Autodesk Inventor part; units mm, degrees
ref_plane "YZ Plane" through (0, 0, 0) normal (1, 0, 0) x (0, 1, 0)
ref_plane "XZ Plane" through (0, 0, 0) normal (0, 1, 0) x (-1, 0, 0)
ref_plane "XY Plane" through (0, 0, 0) normal (0, 0, 1) x (1, 0, 0)
sketch "スケッチ1" plane through (0, 0, 0) normal (0, 1, 0) x (-1, 0, 0)
  line L0 (33.3103, -23) -> (13.3103, -23)
  line L1 (13.3103, -23) -> (-8.6897, -6)
  line L2 (-8.6897, -6) -> (-8.6897, 6)
  line L3 (-8.6897, 6) -> (13.3103, 23)
  line L4 (13.3103, 23) -> (33.3103, 23)
  line L5 (-8.6897, -6) -> (33.3103, 23) construction
  line L6 (33.3103, -23) -> (-8.6897, 6) construction
  line L7 (33.3103, -23) -> (41.3103, -17)
  line L8 (41.3103, -17) -> (41.3103, 17)
  line L9 (41.3103, 17) -> (33.3103, 23)
  point P0 (0, 0)
  point P1 (0, 0)
  dimension "d1" = 46
  dimension "d50" = 20
  dimension "d51" = 20
  dimension "d52" = 17
  dimension "d53" = 17
  dimension "d72" = 8
  dimension "d73" = 6
  dimension "d74" = 6
  dimension "d75" = 50
extrude "押し出し5" add sketch "スケッチ1" along normal blind 5
ref_plane "作業平面2" through (0, 5, 0) normal (0, 1, 0) x (1, 0, 0)
sketch "スケッチ4" plane through (0, 5, 0) normal (0, 1, 0) x (1, 0, 0)
  line L0 (-16.3103, 0) -> (-25.3103, -15.5885)
  line L1 (-25.3103, -15.5885) -> (-16.3103, 0)
  line L2 (-25.3103, 15.5885) -> (-16.3103, 0)
  line L3 (-16.3103, 0) -> (1.6897, 0)
  line L4 (-20.2302, -16.7894) -> (-28.8905, -11.7894)
  line L5 (-28.8905, -11.7894) -> (-30.3905, -14.3875)
  line L6 (-30.3905, -14.3875) -> (-21.7302, -19.3875)
  line L7 (-21.7302, -19.3875) -> (-20.2302, -16.7894)
  line L8 (-20.2302, -16.7894) -> (-30.3905, -14.3875) construction
  line L9 (-28.8905, -11.7894) -> (-21.7302, -19.3875) construction
  line L10 (-20.2302, 16.7894) -> (-28.8905, 11.7894)
  line L11 (-28.8905, 11.7894) -> (-30.3905, 14.3875)
  line L12 (-30.3905, 14.3875) -> (-21.7302, 19.3875)
  line L13 (-21.7302, 19.3875) -> (-20.2302, 16.7894)
  line L14 (-20.2302, 16.7894) -> (-30.3905, 14.3875) construction
  line L15 (-28.8905, 11.7894) -> (-21.7302, 19.3875) construction
  line L16 (-25.2924, -11.5574) -> (-28.7924, -17.6195)
  line L17 (-28.7924, -17.6195) -> (-25.3283, -19.6195)
  line L18 (-25.3283, -19.6195) -> (-21.8283, -13.5574)
  line L19 (-21.8283, -13.5574) -> (-25.2924, -11.5574)
  line L20 (-25.2924, -11.5574) -> (-25.3283, -19.6195) construction
  line L21 (-28.7924, -17.6195) -> (-21.8283, -13.5574) construction
  line L22 (-29.0424, 18.0526) -> (-25.0424, 11.1244)
  line L23 (-25.0424, 11.1244) -> (-21.5783, 13.1244)
  line L24 (-21.5783, 13.1244) -> (-25.5783, 20.0526)
  line L25 (-25.5783, 20.0526) -> (-29.0424, 18.0526)
  line L26 (-29.0424, 18.0526) -> (-21.5783, 13.1244) construction
  line L27 (-25.0424, 11.1244) -> (-25.5783, 20.0526) construction
  line L28 (3.1897, -5) -> (3.1897, 5)
  line L29 (3.1897, 5) -> (0.1897, 5)
  line L30 (0.1897, 5) -> (0.1897, -5)
  line L31 (0.1897, -5) -> (3.1897, -5)
  line L32 (3.1897, -5) -> (0.1897, 5) construction
  line L33 (3.1897, 5) -> (0.1897, -5) construction
  line L34 (5.1897, 2) -> (-1.8103, 2)
  line L35 (-1.8103, 2) -> (-1.8103, -2)
  line L36 (-1.8103, -2) -> (5.1897, -2)
  line L37 (5.1897, -2) -> (5.1897, 2)
  line L38 (5.1897, 2) -> (-1.8103, -2) construction
  line L39 (-1.8103, 2) -> (5.1897, -2) construction
  circle A0 centre (-16.3103, 0) radius 16
  line L40 (-41.3103, 17) -> (-41.3103, -17)
  line L41 (-16.3103, 0) -> (-34.3103, 0)
  line L42 (-32.8103, -5) -> (-35.8103, -5)
  line L43 (-35.8103, -5) -> (-35.8103, 5)
  line L44 (-35.8103, 5) -> (-32.8103, 5)
  line L45 (-32.8103, 5) -> (-32.8103, -5)
  line L46 (-32.8103, -5) -> (-35.8103, 5) construction
  line L47 (-35.8103, -5) -> (-32.8103, 5) construction
  line L48 (-38.3103, -2) -> (-30.3103, -2)
  line L49 (-30.3103, -2) -> (-30.3103, 2)
  line L50 (-30.3103, 2) -> (-38.3103, 2)
  line L51 (-38.3103, 2) -> (-38.3103, -2)
  line L52 (-38.3103, -2) -> (-30.3103, 2) construction
  line L53 (-30.3103, -2) -> (-38.3103, 2) construction
  point P0 (-31.7241, 0)
  point P1 (-41.3103, 0)
  point P2 (-41.3103, 0)
  dimension "d8" = 120
  dimension "d9" = 120
  dimension "d10" = 18
  dimension "d11" = 18
  dimension "d12" = 18
  dimension "d13" = 4
  dimension "d14" = 4
  dimension "d15" = 4
  dimension "d16" = 7
  dimension "d17" = 3
  dimension "d18" = 10
  dimension "d19" = 8
  dimension "d20" = 10
  dimension "d21" = 3
  dimension "d22" = 10
  dimension "d23" = 3
  dimension "d24" = 7
  dimension "d29" = 32
  dimension "d79" = 25
  dimension "d121" = 18
  dimension "d122" = 4
  dimension "d123" = 8
  dimension "d124" = 3
  dimension "d125" = 10
extrude "押し出し2" cut sketch "スケッチ4" against normal blind 10 contours L19 L18 A0 L0 | L0 A0 L16 L19 | L23 L22 A0 L2 | L2 A0 L24 L23 | L35 L34 A0 L3 | L3 A0 L36 L35 | L49 L48 A0 L41 | L41 A0 L50 L49 | A0 L18 L4 L0 | L0 L4 L16 A0 | A0 L22 L10 L2 | L2 L10 L24 A0 | A0 L34 L30 L3 | L3 L30 L36 A0 | L41 L45 L50 A0 | A0 L48 L45 L41 | L4 L18 L6 L16 | L10 L22 L12 L24 | L30 L34 L28 L36 | L45 L48 L43 L50 | L18 L17 L16 L6 | L12 L22 L25 L24 | L34 L37 L36 L28 | L43 L48 L51 L50
extrude "押し出し3" cut sketch "スケッチ4" against normal blind 3 contours L4 L18 L6 L16 | L10 L22 L12 L24 | L30 L34 L28 L36 | L45 L48 L43 L50 | L4 L7 L6 L18 | L16 L6 L5 L4 | L24 L12 L13 L10 | L10 L11 L12 L22 | L30 L29 L28 L34 | L36 L28 L31 L30 | L50 L43 L44 L45 | L45 L42 L43 L48
extrude "押し出し4" cut sketch "スケッチ4" against normal blind 10 contours L3 L35 L36 A0 L18 L19 L0 | L41 L49 L50 A0 L22 L23 L2 | L2 L23 L24 A0 L34 L35 L3 | L0 L19 L16 A0 L48 L49 L41 | L19 L18 A0 L0 | L0 A0 L16 L19 | L23 L22 A0 L2 | L2 A0 L24 L23 | L35 L34 A0 L3 | L3 A0 L36 L35 | L49 L48 A0 L41 | L41 A0 L50 L49
ref_plane "作業平面1" through (0, 5, 0) normal (0, 1, 0) x (1, 0, 0)
sketch "スケッチ6" plane through (0, 5, 0) normal (0, 1, 0) x (1, 0, 0)
  line L0 (8.6897, -6) -> (8.6897, 6)
  line L1 (-33.3103, -23) -> (-13.3103, -23)
  line L2 (-13.3103, 23) -> (-33.3103, 23)
  point P0 (0, 0)
  point P1 (5.6897, 5)
  point P2 (5.6897, -5)
  point P3 (-37.3103, 13)
  point P4 (-37.3103, -13)
  dimension "d58" = 1
  dimension "d59" = 1
  dimension "d60" = 24
  dimension "d80" = 3
  dimension "d81" = 10
  dimension "d82" = 10
hole "穴2" at (5.6897, 5, -5) at (5.6897, 5, 5) at (-37.3103, 5, -13) at (-37.3103, 5, 13) direction (0, -1, 0) diameter 3 end through all
equation "\"d11\" = d10"
equation "\"d12\" = d10"
equation "\"d14\" = d13"
equation "\"d15\" = d13"
equation "\"d20\" = d18"
equation "\"d21\" = d17"
equation "\"d22\" = d18"
equation "\"d23\" = d17"
equation "\"d24\" = d16"
equation "\"d121\" = d11"
equation "\"d122\" = d14"
equation "\"d123\" = d19"
equation "\"d124\" = d21"
equation "\"d125\" = d20"
equation "\"d66\" = Thickness"
equation "\"BendRadius\" = Thickness"
equation "\"BendReliefWidth\" = Thickness"
equation "\"BendReliefDepth\" = 0.5 * Thickness"
equation "\"TransitionRadius\" = BendRadius"
equation "\"JacobiRadiusSize\" = Thickness"
equation "\"GapSize\" = Thickness"
equation "\"d2\" = Thickness"
properties part number "trackball-base" material "アルミニウム 6061"
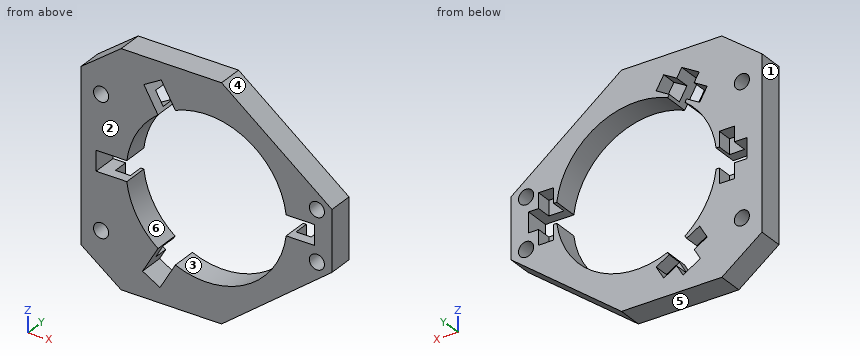
Design review of the part built by this model. Coordinates are the model's own, in mm. Face numbers are marked on the shaded views. A direction names the side the tool comes from. Give positions to 0.01 mm unless a question says otherwise; leave off trailing zeros. Loops run counter-clockwise (first coordinate to the right, second up) from the corner with the lowest first, then second, coordinate; pieces in that order, holes last. Notation, with made-up numbers: (-24.5, 70.5) - (-18.5, 70.5) arc R23 cw to (-18.5, 82.5) - close; hole circle Ø7 at (-29, 68). An arc over 180 degrees is marked (long way). Use CSV: the item, a comma, the result in double quotes. Start each with the question number.
1. Machinability: for the marked faces 5 and 6, which of the approach directions +Z, -Z, +X, -X, +Y, -Y give a long, thin tool a straight path to every point of the face, cutting with its end or side? Answer none if there is none.
2. Draft analysis for pull direction X (two halves, no side actions). For the marked faces 1, 2, 3 and 4, state which applies: released by +X, released by -X, zero draft, split by the parting line, or undercut.
3. Insertion check: P1, Ø1.5, axis at x = -1, y = 1.5, coming from the +Z side; P2, Ø3.5, axis at x = -34, z = -3.5, coming from the +Y side; P3, Ø2.5, axis at x = 2, y = 3, coming from the +Z side; P4, Ø1.5, axis at x = 2, z = 4, coming from the +Y side. Each pin has a flat end and moves straight along its axis. Give the tip position at first contact, or say it passes through.
4. Add section C-C (y = 0.6). State the section outline as (x, z) points, plus the area to 3 significant figures.
5. Add section D-D (x = -19). State the section outline as (y, z) points, plus the area to 3 significant figures.
6. Wall thickness on L1, parallel to X at y = 3.7, z = -4; L2, parallel to Z at x = -21, y = 4; L3, parallel to X at y = 4.55, z = -12 (3 decimals): over which ranges is each line inside the solid? List them lowest first.
7. Add section B-B (x = -27). State the section outline as (y, z) points.
8. Add section A-A (z = -0.5). State the section outline as (x, y) points.
Results found:
1,face 5,"-Z, +X, -X, +Y, -Y"
1,face 6,"+Y, -Y"
2,face 1,"released by -X"
2,face 2,"zero draft"
2,face 3,"undercut"
2,face 4,"released by +X"
3,P1,"stops at z = 14.07"
3,P2,"stops at y = 5"
3,P3,"stops at z = 12.14"
3,P4,"stops at y = 2"
4,outline,"(-41.31, -17) - (-33.31, -23) - (-13.31, -23) - (8.69, -6) - (8.69, 6) - (-13.31, 23) - (-33.31, 23) - (-41.31, 17) - close; hole circle Ø3 at (-37.31, -13); hole circle Ø3 at (-37.31, 13); hole (-38.31, -2) - (-32.18, -2) arc R16 ccw to (-25.98, -12.75) - (-29.04, -18.05) - (-25.58, -20.05) - (-22.52, -14.75) arc R16 ccw to (-0.44, -2) - (5.19, -2) - (5.19, 2) - (-0.44, 2) arc R16 ccw to (-22.52, 14.75) - (-25.33, 19.62) - (-28.79, 17.62) - (-25.98, 12.75) arc R16 ccw to (-32.18, 2) - (-38.31, 2) - close; hole circle Ø3 at (5.69, -5); hole circle Ø3 at (5.69, 5)"
4,area,"953 mm²"
5,outline,"(0, -23) - (5, -23) - (5, -15.77) - (0, -15.77) - close; (0, 15.77) - (5, 15.77) - (5, 23) - (0, 23) - close"
5,area,"72.3 mm²"
6,L1,"x = -41.31 to -35.81, -32.81 to -31.8, -0.82 to 0.19, 3.19 to 4.57, 6.81 to 8.69"
6,L2,"z = -23 to -18.12, -16.34 to -15.3, 15.3 to 16.34, 18.12 to 23"
6,L3,"x = -41.31 to -38.428, -36.192 to -29.012, -28.526 to -26.893, -5.727 to 0.925"
7,outline,"(0, -23) - (5, -23) - (5, -19.23) - (0, -19.23) - close; (0, -14.52) - (2, -14.52) - (2, -12.88) - (5, -12.88) - (5, -11.91) - (0, -11.91) - close; (0, 11.91) - (5, 11.91) - (5, 12.88) - (2, 12.88) - (2, 14.52) - (0, 14.52) - close; (0, 18.65) - (5, 18.65) - (5, 23) - (0, 23) - close"
8,outline,"(-41.31, 0) - (-38.31, 0) - (-38.31, 5) - (-41.31, 5) - close; (5.19, 0) - (8.69, 0) - (8.69, 5) - (5.19, 5) - close"
